Autodesk Inventor part; units mm, degrees
ref_plane "YZ Plane" through (0, 0, 0) normal (1, 0, 0) x (0, 1, 0)
ref_plane "XZ Plane" through (0, 0, 0) normal (0, 1, 0) x (-1, 0, 0)
ref_plane "XY Plane" through (0, 0, 0) normal (0, 0, 1) x (1, 0, 0)
sketch "Sketch1" plane through (0, 0, 0) normal (0, 0, 1) x (1, 0, 0)
  circle A0 centre (0, 0) radius 7.5
  circle A1 centre (-35, 0) radius 4
  line L0 (-35.4, 3.9799) -> (-0.75, 7.4624)
  line L1 (-0.75, -7.4624) -> (-35.4, -3.9799)
  dimension "d0" = 15
  dimension "d1" = 8
  dimension "d2" = 35
extrude "Extrusion1" add sketch "Sketch1" along normal blind 3
sketch "Sketch3" plane through (0, 0, 3) normal (0, 0, 1) x (1, 0, 0)
  arc A0 (-35.4, 3.9799) -> (-35.4, -3.9799) centre (-35, 0) ccw
  line L0 (-35.4, -3.9799) -> (-0.75, -7.4624)
  arc A1 (-0.75, -7.4624) -> (-0.75, 7.4624) centre (0, 0) ccw
  line L1 (-0.75, 7.4624) -> (-35.4, 3.9799)
hole "Hole1" at (0, 0, 3) direction (0, 0, -1) diameter 5.5 end through all
sketch "Sketch4" plane through (0, 0, 3) normal (0, 0, 1) x (1, 0, 0)
  circle A0 centre (0, 0) radius 2.75
  arc A1 (-35.4, 3.9799) -> (-35.4, -3.9799) centre (-35, 0) ccw
  line L0 (-35.4, -3.9799) -> (-0.75, -7.4624)
  arc A2 (-0.75, -7.4624) -> (-0.75, 7.4624) centre (0, 0) ccw
  line L1 (-0.75, 7.4624) -> (-35.4, 3.9799)
hole "Hole2" at (-35, 0, 3) direction (0, 0, -1) diameter 3.4 end through all
properties part number "Selection_Counterweight" material "Nylon 6/6"
Design review of the part built by this model. Coordinates are the model's own, in mm. Coordinates: 2 decimals unless noted, no trailing zeros. Order: outer loops, then holes, each group sorted by start corner. A loop starts at its lowest first (then second) coordinate and runs counter-clockwise, first axis right, second up. Notation, with made-up numbers: (43, 23.5) -> (47, 23.5) arc R22 ccw to (47, 29.5) -> close; hole circle Ø7 at (68.5, -20.5). An arc over 180 degrees is marked (long way). Use one line per item in the form item = value. Start each with the question number.
(1) Add section C-C on z = 0.9. State the section outline as (x, y) points, plus the area to 3 significant figures.
(2) Add section A-A on y = 0. State the section outline as (x, z) points.
(3) The part is to be moulded in two halves that separate along X. For faces 1 (the flat face through (-16, 0, 3)), 2 (the cylindrical face through (-33.34, 0.37, 1.48)), 3 (the flat face through (-17.832, -5.746, 1.479)), say which applies: +X half, -X half, draft (parallel to the pull), parting line (faces both ways), or undercut.
(4) Insertion check: pin 1 (4.5 mm diameter, centred on x = 0, y = 0, fed in from -Z). The pin has a flat end and moves straight along its axis. Give the tip position at first contact, or say it passes through.
(5) Add section D-D on x = -35. State the section outline as (y, z) points, plus the area to 3 significant figures.
(6) For probe 1 along X at (y, z) = (0, 1.9); probe 2 along Y at (x, z) = (0, 2.45); probe 3 along X at (y, z) = (-1.25, 1.75), list the stretches that pass through material, from the lowest coordinate up.
(7) Add section B-B on x = 0. State the section outline as (y, z) points.
Answer block:
q1.outline = (-35.4, -3.98) -> (-0.75, -7.46) arc R7.5 ccw (long way) to (-0.75, 7.46) -> (-35.4, 3.98) arc R4 ccw to start; hole circle Ø3.4 at (-35, 0); hole circle Ø5.5 at (0, 0)
q1.area = 485 mm²
q2.outline = (-39, 0) -> (-36.7, 0) -> (-36.7, 3) -> (-39, 3) -> close; (-33.3, 0) -> (-2.75, 0) -> (-2.75, 3) -> (-33.3, 3) -> close; (2.75, 0) -> (7.5, 0) -> (7.5, 3) -> (2.75, 3) -> close
q3.face_1 = draft
q3.face_2 = undercut
q3.face_3 = -X half
q4.pin_1 = through
q5.outline = (-4.02, 0) -> (-1.7, 0) -> (-1.7, 3) -> (-4.02, 3) -> close; (1.7, 0) -> (4.02, 0) -> (4.02, 3) -> (1.7, 3) -> close
q5.area = 13.9 mm²
q6.probe_1 = -39 to -36.7, -33.3 to -2.75, 2.75 to 7.5
q6.probe_2 = -7.5 to -2.75, 2.75 to 7.5
q6.probe_3 = -38.8 to -36.15, -33.85 to -2.45, 2.45 to 7.4
q7.outline = (-7.5, 0) -> (-2.75, 0) -> (-2.75, 3) -> (-7.5, 3) -> close; (2.75, 0) -> (7.5, 0) -> (7.5, 3) -> (2.75, 3) -> close
